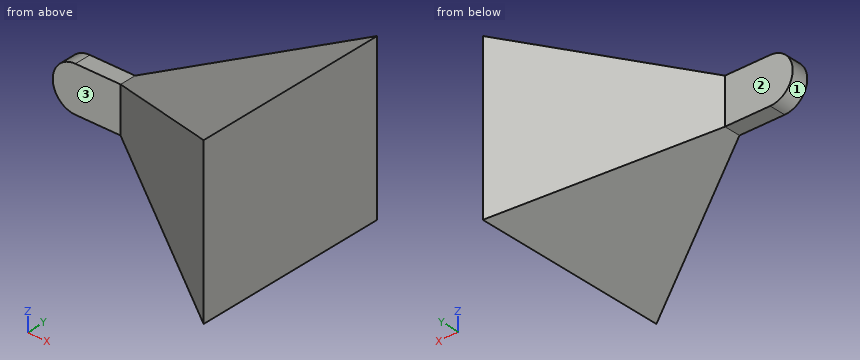
```python
from build123d import *

# Parameters (mm, degrees)
BOSS_EXTRUDE1_DEPTH      = 139.7
BOSS_EXTRUDE1_DEPTH_BACK = 139.7
CUT_EXTRUDE1_DEPTH       = 139.7
CUT_EXTRUDE1_DEPTH_BACK  = 139.7


with BuildPart() as part:
    # Sketch1 → Boss-Extrude1 (new, two sides: drawn at the far end of the back side and taken through both)
    with BuildSketch(Plane(origin=(0, 0, 0), x_dir=(1, 0, 0), z_dir=(0, 1, 0)).offset(-BOSS_EXTRUDE1_DEPTH_BACK)):
        with BuildLine():
            Line((0, 31.75), (63.5, 31.75))
            Line((63.5, 31.75), (292.1, 114.3))
            Line((292.1, 114.3), (292.1, -114.3))
            Line((292.1, -114.3), (63.5, -31.75))
            Line((63.5, -31.75), (0, -31.75))
            ThreePointArc((0, -31.75), (-31.75, 0), (0, 31.75))
        make_face()
    extrude(amount=BOSS_EXTRUDE1_DEPTH + BOSS_EXTRUDE1_DEPTH_BACK)

    # Sketch2 → Cut-Extrude1 (cut, two sides: drawn at the far end of the back side and taken through both)
    with BuildSketch(Plane.XY.offset(-CUT_EXTRUDE1_DEPTH_BACK)):
        Polygon((-31.75, 11.723949014), (63.5, 11.723949014), (292.1, 139.7), (-31.75, 139.7), align=None)
        Polygon((63.5, -11.723949014), (292.1, -139.7), (-31.75, -139.7), (-31.75, -11.723949014), align=None)
    extrude(amount=CUT_EXTRUDE1_DEPTH + CUT_EXTRUDE1_DEPTH_BACK, mode=Mode.SUBTRACT)


solid = part.part
```
The model under review builds one solid part; all positions refer to its coordinate system, in mm. Face numbers are marked on the shaded views. A direction names the side the tool comes from. Give positions to 0.01 mm unless a question says otherwise; leave off trailing zeros. Write each loop counter-clockwise with the first axis right and the second up, starting at its lowest first coordinate (ties: lowest second). Pieces come first, ordered by that corner, then holes.
(1) To check wall thickness, follow L1, parallel to Y at x = 20.5, z = 1.5; L2, parallel to Z at x = 37, y = -7.5; L3, parallel to Y at x = 183, z = 61. State the ranges of each line that lie inside material, in increasing order.
(2) Consider section C-C, the plane y = -33. Give the boundary of the cut face in (x, z).
(3) Tool access review of the marked faces 1, 2 and 3: name each direction out of +Z, -Z, +X, -X, +Y, -Y from which nothing blocks a thin tool from reaching the whole face with its end or side.
(4) Consider section B-B, the plane x = 34.5. Give the boundary of the cut face in (y, z), and give its area (3 significant figures).
(5) Consider section A-A, the plane z = 0. Give the boundary of the cut face in (x, y).
(6) For P1, Ø3, axis at y = 101, z = -81, coming from the -X side; P2, Ø6, axis at x = 157.5, z = 19, coming from the +Y side; P3, Ø1, axis at x = 118, y = -20, coming from the +Z side, all flat-tipped, find the tip position at first contact; note any pin that passes through.
Returned:
1. L1: y = -11.72 to 11.72
1. L2: z = -31.75 to 31.75
1. L3: y = -78.62 to 78.62
2. outline: (101.5, -45.47) - (292.1, -114.3) - (292.1, 114.3) - (101.5, 45.47) - close
3. face 1: -X, +Y, -Y
3. face 2: +Z, -Z, -X, +Y
3. face 3: +Z, -Z, -X, -Y
4. outline: (-11.72, -31.75) - (11.72, -31.75) - (11.72, 31.75) - (-11.72, 31.75) - close
4. area: 1,490 mm2
5. outline: (-31.75, -11.72) - (63.5, -11.72) - (292.1, -139.7) - (292.1, 139.7) - (63.5, 11.72) - (-31.75, 11.72) - close
6. P1: stops at x = 220.29
6. P2: stops at y = 66.03
6. P3: stops at z = 51.61
